The model under review builds one solid part; all positions refer to its coordinate system, in mm. Round coordinates to 2 decimals unless told otherwise and drop trailing zeros. Write each loop counter-clockwise with the first axis right and the second up, starting at its lowest first coordinate (ties: lowest second). Pieces come first, ordered by that corner, then holes. Notation, with made-up numbers: M 49,88.5 L 98,88.5 A23 ccw 98,96.5 Z; hole C -16.5,77 d3. An arc over 180 degrees is marked long. Write item = value, one per line. Start each with the question number.
Item 1: Take a section at A-A, the plane y = -36. Give the boundary of the cut face in (x, z), plus the area to 3 significant figures.
Item 2: For pin 1 Ø4.5 at (x, y) = (5, -36) entering from -Z; pin 2 Ø2.5 at (x, y) = (-5, -36) entering from +Z; pin 3 Ø1 at (y, z) = (6, 2) entering from -X; pin 4 Ø1.5 at (y, z) = (-48.5, 1.5) entering from +X (3 decimals), all flat-tipped, find the tip position at first contact; note any pin that passes through.
Item 3: Take a section at B-B, the plane y = -6. Give the boundary of the cut face in (x, z).
Item 4: Take a section at D-D, the plane x = 5. Give the boundary of the cut face in (y, z).
Item 5: To check wall thickness, follow line 1 along X through (y, z) = (-25.5, 1.1); line 2 along Y through (x, z) = (-5, 1.2); line 3 along Y through (x, z) = (-8.5, 0.8). State the ranges of each line that lie inside material, in increasing order.
Item 6: Take a section at C-C, the plane z = 1.9. Give the boundary of the cut face in (x, y) (3 decimals).
from build123d import *

# Parameters (mm, degrees)
CROQUIS1_R              = 2
CROQUIS1_W              = 20.3
CROQUIS1_H              = 40.3
SALIENTE_EXTRUIR1_DEPTH = 3


with BuildPart() as part:
    # Croquis1 → Saliente-Extruir1 (new body)
    with BuildSketch(Plane.XY):
        with BuildLine():
            Line((40, 0), (40, -47))
            Line((40, -47), (20.175, -47))
            Line((20.175, -47), (20.175, -50.2))
            Line((20.175, -50.2), (-20.175, -50.2))
            Line((-20.175, -50.2), (-20.175, -47))
            Line((-20.175, -47), (-40, -47))
            Line((-40, -47), (-40, 0))
            ThreePointArc((-40, 0), (-28.284271247, 28.284271247), (0, 40))
            ThreePointArc((0, 40), (28.284271247, 28.284271247), (40, 0))
        make_face()
        with Locations((-5, 12.3)):
            Circle(CROQUIS1_R, mode=Mode.SUBTRACT)
        with Locations(Location((5, 12.3, 0), (0, 0, 180))):
            Circle(CROQUIS1_R, mode=Mode.SUBTRACT)
        with Locations((5, -36)):
            Circle(CROQUIS1_R, mode=Mode.SUBTRACT)
        with Locations(Location((-5, -36, 0), (0, 0, 180))):
            Circle(CROQUIS1_R, mode=Mode.SUBTRACT)
        with Locations((-30, -11.85)):
            Circle(CROQUIS1_R, mode=Mode.SUBTRACT)
        with Locations(Location((30, -11.85, 0), (0, 0, 180))):
            Circle(CROQUIS1_R, mode=Mode.SUBTRACT)
        with Locations((0, -11.85)):
            Rectangle(CROQUIS1_W, CROQUIS1_H, mode=Mode.SUBTRACT)
    extrude(amount=SALIENTE_EXTRUIR1_DEPTH)


solid = part.part
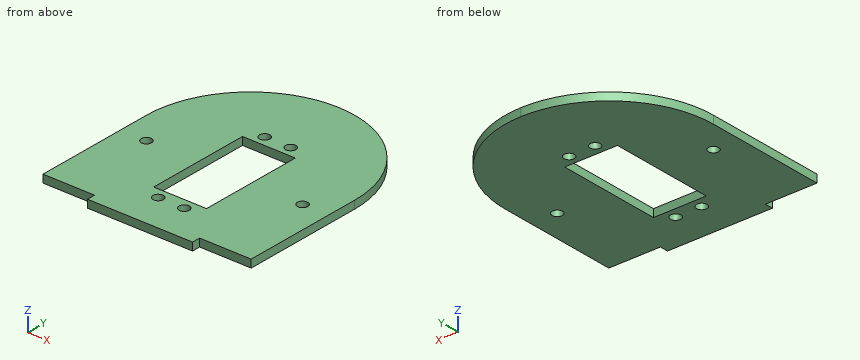
Response values:
q1.outline = M -40,0 L -7,0 L -7,3 L -40,3 Z; M -3,0 L 3,0 L 3,3 L -3,3 Z; M 7,0 L 40,0 L 40,3 L 7,3 Z
q1.area = 216 mm2
q2.pin_1 = 0
q2.pin_2 = through
q2.pin_3 = -39.62
q2.pin_4 = 20.175
q3.outline = M -40,0 L -10.15,0 L -10.15,3 L -40,3 Z; M 10.15,0 L 40,0 L 40,3 L 10.15,3 Z
q4.outline = M -50.2,0 L -38,0 L -38,3 L -50.2,3 Z; M -34,0 L -32,0 L -32,3 L -34,3 Z; M 8.3,0 L 10.3,0 L 10.3,3 L 8.3,3 Z; M 14.3,0 L 39.69,0 L 39.69,3 L 14.3,3 Z
q5.line_1 = -40 to -10.15, 10.15 to 40
q5.line_2 = -50.2 to -38, -34 to -32, 8.3 to 10.3, 14.3 to 39.69
q5.line_3 = -50.2 to -32, 8.3 to 39.09
q6.outline = M -40,-47 L -20.175,-47 L -20.175,-50.2 L 20.175,-50.2 L 20.175,-47 L 40,-47 L 40,0 A40 ccw -40,0 Z; hole C -30,-11.85 d4; hole M -10.15,-32 L 10.15,-32 L 10.15,8.3 L -10.15,8.3 Z; hole C -5,-36 d4; hole C -5,12.3 d4; hole C 5,-36 d4; hole C 5,12.3 d4; hole C 30,-11.85 d4
